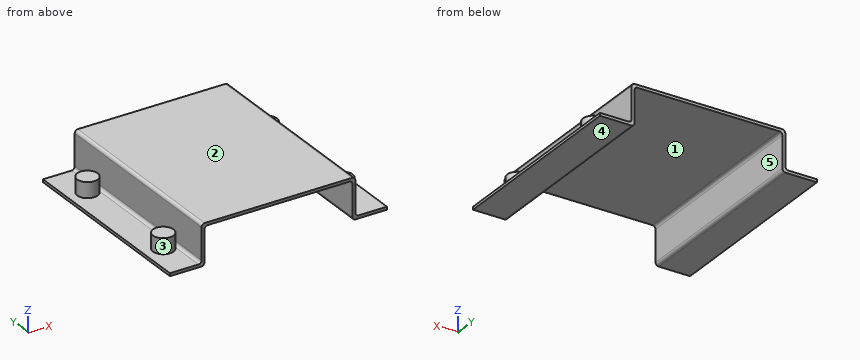
```python
from build123d import *

# Parameters (mm, degrees)
F1_DEPTH = 77
F2_R     = 1.2
F3_R     = 4
F4_DEPTH = 6


with BuildPart() as f1:
    # F0 (on Front) → F1 (new body)
    with BuildSketch(Plane.XZ):
        Polygon((-42.38, 1.12), (-42.38, 0), (-28.88, 0), (-28.88, 14.755), (28.88, 14.755), (28.88, 0), (42.38, 0), (42.38, 1.12), (30, 1.12), (30, 15.875), (-30, 15.875), (-30, 1.12), align=None)
    extrude(amount=F1_DEPTH)

    # F2
    f2_edges = [f1.edges().sort_by_distance(p)[0] for p in [
        (-30, -38.5, 15.875),
        (30, -38.5, 15.875),
        (28.88, -38.5, 0),
        (-28.88, -38.5, 0),
        (28.88, -38.5, 14.755),
        (-28.88, -38.5, 14.755),
        (-30, -38.5, 1.12),
        (30, -38.5, 1.12),
    ]]
    fillet(f2_edges, radius=F2_R)

    # F3 (on face) → F4 (join)
    with BuildSketch(Plane.XY.offset(1.12)):
        with Locations((35, -15.5)):
            Circle(F3_R)
        with Locations((35, -61.5)):
            Circle(F3_R)
        with Locations((-35, -15.5)):
            Circle(F3_R)
        with Locations((-35, -61.5)):
            Circle(F3_R)
    extrude(amount=F4_DEPTH)


solid = f1.part
```
Verification items for the finished model (mm, model axes). Face numbers are marked on the shaded views. A direction names the side the tool comes from. Round coordinates to 2 decimals unless told otherwise and drop trailing zeros. Order: outer loops, then holes, each group sorted by start corner. A loop starts at its lowest first (then second) coordinate and runs counter-clockwise, first axis right, second up. Notation, with made-up numbers: (-20.75, -35.75) - (34.25, -35.75) arc R11 cw to (34.25, -25.75) - close; hole circle Ø11 at (56, 25.5). An arc over 180 degrees is marked (long way). Use CSV: the item, a comma, the result in double quotes. Start each with the question number.
1) Section check A-A, the plane z = 3.75. Record the cut outline in (x, y).
2) Access from +Z, -Z, +X, -X, +Y, -Y to the whole of each face (thin tool, end or side, straight path). Record for the marked faces 3, 4 and 5.
3) Mould release check, pull along X, two halves, no side actions. Record for the marked faces 1 and 2: +X half, -X half, draft (parallel to the pull), parting line (faces both ways), or undercut.
4) Go/stop test with flat-tipped pins: P1, Ø6.5, axis at x = -35.5, y = -59.5, coming from the +Z side; P2, Ø6, axis at y = -45, z = 7.5, coming from the +X side; P3, Ø12.5, axis at x = 34.5, y = -45.5, coming from the +Z side (3 decimals); P4, Ø1.5, axis at x = 11.5, y = -35.5, coming from the -Z side (3 decimals). Record where each tip stops, or that it passes through.
5) Thickness scan on L1, parallel to X at y = -22, z = 5; L2, parallel to X at y = -14, z = 1.25; L3, parallel to Z at x = 36.5, y = -58. Record the ranges inside material, lowest first.
6) Section check D-D, the plane x = -20. Record the cut outline in (y, z) (3 decimals), plus the area to 3 significant figures.
7) Section check C-C, the plane x = 35. Record the cut outline in (y, z), plus the area to 3 significant figures.
8) Section check B-B, the plane y = -50.5. Record the cut outline in (x, z) (3 decimals), plus the area to 3 significant figures.
Answers:
1,outline,"circle Ø8 at (-35, -61.5); circle Ø8 at (-35, -15.5); (-30, -77) - (-28.88, -77) - (-28.88, 0) - (-30, 0) - close; (28.88, -77) - (30, -77) - (30, 0) - (28.88, 0) - close; circle Ø8 at (35, -61.5); circle Ø8 at (35, -15.5)"
2,face 3,"+Z"
2,face 4,"-Z, +X, -X, +Y, -Y"
2,face 5,"-Z, +Y, -Y"
3,face 1,"undercut"
3,face 2,"draft"
4,P1,"stops at z = 7.12"
4,P2,"stops at x = 30"
4,P3,"stops at z = 15.875"
4,P4,"stops at z = 14.755"
5,L1,"x = -30 to -28.88, 28.88 to 30"
5,L2,"x = -38.71 to -31.29, -30.66 to -28.88, 28.88 to 30.66, 31.29 to 38.71"
5,L3,"z = 0 to 7.12"
6,outline,"(-77, 14.755) - (0, 14.755) - (0, 15.875) - (-77, 15.875) - close"
6,area,"86.2 mm²"
7,outline,"(-77, 0) - (0, 0) - (0, 1.12) - (-11.5, 1.12) - (-11.5, 7.12) - (-19.5, 7.12) - (-19.5, 1.12) - (-57.5, 1.12) - (-57.5, 7.12) - (-65.5, 7.12) - (-65.5, 1.12) - (-77, 1.12) - close"
7,area,"182 mm²"
8,outline,"(-42.38, 0) - (-30.08, 0) arc R1.2 ccw to (-28.88, 1.2) - (-28.88, 13.555) arc R1.2 cw to (-27.68, 14.755) - (27.68, 14.755) arc R1.2 cw to (28.88, 13.555) - (28.88, 1.2) arc R1.2 ccw to (30.08, 0) - (42.38, 0) - (42.38, 1.12) - (31.2, 1.12) arc R1.2 cw to (30, 2.32) - (30, 14.675) arc R1.2 ccw to (28.8, 15.875) - (-28.8, 15.875) arc R1.2 ccw to (-30, 14.675) - (-30, 2.32) arc R1.2 cw to (-31.2, 1.12) - (-42.38, 1.12) - close"
8,area,"128 mm²"
